```python
from build123d import *

# Parameters (mm, degrees)
BOSS_EXTRUDE1_DEPTH = 250
BOSS_EXTRUDE6_DEPTH = 125
BOSS_EXTRUDE7_DEPTH = 125


with BuildPart() as part:
    # Sketch1 → Boss-Extrude1 (new body)
    with BuildSketch(Plane(origin=(0, 0, 0), x_dir=(0, 0, -1), z_dir=(1, 0, 0))):
        with BuildLine():
            Line((-10, 7.5), (10, 7.5))
            ThreePointArc((10, 7.5), (17.5, 0), (10, -7.5))
            Line((10, -7.5), (-10, -7.5))
            ThreePointArc((-10, -7.5), (-17.5, 0), (-10, 7.5))
        make_face()
    extrude(amount=BOSS_EXTRUDE1_DEPTH)

    # Sketch11 → Boss-Extrude6 (add)
    with BuildSketch(Plane(origin=(0, 7.5, 0), x_dir=(1, 0, 0), z_dir=(0, 1, 0))):
        with BuildLine():
            Line((1.220843579, -10), (1.220843579, 10))
            ThreePointArc((1.220843579, 10), (8.447072594, 17.226229015), (15.673301609, 10))
            Line((15.673301609, 10), (15.673301609, -10))
            ThreePointArc((15.673301609, -10), (8.447072594, -17.226229015), (1.220843579, -10))
        make_face()
    extrude(amount=BOSS_EXTRUDE6_DEPTH)

    # Sketch12 → Boss-Extrude7 (add)
    with BuildSketch(Plane(origin=(-58.413349195, 58.413349195, 0), x_dir=(-0.7071067811865476, -0.7071067811865476, 0), z_dir=(0.7071067811865476, -0.7071067811865476, 0))):
        with BuildLine():
            Line((-105.56811993, -15), (-105.56811993, 15))
            ThreePointArc((-105.56811993, 15), (-100.022563681, 20.545556249), (-94.477007433, 15))
            Line((-94.477007433, 15), (-94.477007433, -15))
            ThreePointArc((-94.477007433, -15), (-100.022563681, -20.545556249), (-105.56811993, -15))
        make_face()
    extrude(amount=-BOSS_EXTRUDE7_DEPTH)


solid = part.part
```
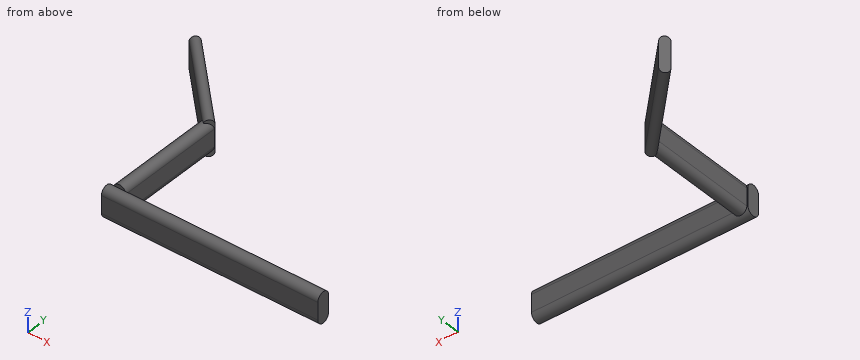
Geometry: final body of the model. Coordinates: model frame, mm. Round coordinates to 2 decimals unless told otherwise and drop trailing zeros. Order: outer loops, then holes, each group sorted by start corner. A loop starts at its lowest first (then second) coordinate and runs counter-clockwise, first axis right, second up. Notation, with made-up numbers: (-10.5, 69) -> (-4.5, 69) arc R21 cw to (-4.5, 79) -> close; hole circle Ø3 at (77.25, 87.25). An arc over 180 degrees is marked (long way). Use CSV: the item, a comma, the result in double quotes. Start each with the question number.
1) Material intervals for line 1 along Y through (x, z) = (121, 3); line 2 along X through (y, z) = (124.5, -8); line 3 along X through (y, z) = (155.5, 17), sorted ascending. Write a range as from..to.
2) First-contact query: pin 1 Ø2 at (y, z) = (46, 14.5) entering from -X (3 decimals); pin 2 Ø5 at (y, z) = (122.5, -8.5) entering from -X; pin 3 Ø2 at (y, z) = (30, -10.5) entering from +X. Flat tips, straight axial feed; report the tip coordinate or a pass-through.
3) Section C-C (y = 0). Return the cut outline in (x, z), and give its area (3 significant figures).
4) Section A-A (z = 1). Return the cut outline in (x, y).
5) Section B-B (x = 60.5). Return the cut outline in (y, z).
Returned:
1,line 1,"y = -7.5..7.5"
1,line 2,"x = 1.22..15.67"
1,line 3,"x = -21.36..-6.73"
2,pin 1,"stops at x = 2.125"
2,pin 2,"stops at x = 1.22"
2,pin 3,"stops at x = 15.67"
3,outline,"(0, -17.5) -> (250, -17.5) -> (250, 17.5) -> (0, 17.5) -> close"
3,area,"8,750 mm²"
4,outline,"(-80, 213.61) -> (1.22, 132.39) -> (1.22, 7.5) -> (0, 7.5) -> (0, -7.5) -> (250, -7.5) -> (250, 7.5) -> (15.67, 7.5) -> (15.67, 132.5) -> (16.23, 133.06) -> (-72.15, 221.45) -> close"
5,outline,"(-7.5, -10) arc R7.5 ccw to (7.5, -10) -> (7.5, 10) arc R7.5 ccw to (-7.5, 10) -> close"
